```python
from build123d import *

# Parameters (mm, degrees)
ESQUISSE1_W                  = 65
ESQUISSE1_H                  = 30
BOSS_EXTRU_1_DEPTH           = 2
ESQUISSE2_R                  = 3
BOSS_EXTRU_2_DEPTH           = 8
BOSS_EXTRU_2_DRAFT           = 18
BOSS_EXTRU_2_PROFILE_2_DEPTH = 8
BOSS_EXTRU_2_PROFILE_2_DRAFT = 18
BOSS_EXTRU_2_PROFILE_3_DEPTH = 8
BOSS_EXTRU_2_PROFILE_3_DRAFT = 18
BOSS_EXTRU_2_PROFILE_4_DEPTH = 8
BOSS_EXTRU_2_PROFILE_4_DRAFT = 18
ENL_V_MAT_EXTRU_2_REACH      = 41.058
ESQUISSE4_W                  = 22.5
ESQUISSE4_H                  = 14
ENL_V_MAT_EXTRU_3_REACH      = 41.058
ESQUISSE5_R                  = 1.5
CONG_1_R                     = 2
BOSS_EXTRU_3_REACH           = 41.415
ENL_V_MAT_EXTRU_4_REACH      = 41.415
ESQUISSE7_R                  = 1.2


with BuildPart() as part:
    # Esquisse1 → Boss.-Extru.1 (new body)
    with BuildSketch(Plane.XY):
        Rectangle(ESQUISSE1_W, ESQUISSE1_H)
    extrude(amount=BOSS_EXTRU_1_DEPTH)


with BuildPart() as boss_extru_2_tool:
    # Esquisse2 → Boss.-Extru.2 (with draft: the straight prism first)
    with BuildSketch(Plane.XY.offset(8)):
        with Locations((-29, 11.5)):
            Circle(ESQUISSE2_R)
    extrude(amount=-BOSS_EXTRU_2_DEPTH)
    # Boss.-Extru.2: the draft: its side faces are tilted about the plane it starts from
    boss_extru_2_sides = [boss_extru_2_tool.faces().sort_by_distance(p)[0] for p in [
        (-32, 11.5, 4),
    ]]
    draft(boss_extru_2_sides, Plane.XY.offset(8), BOSS_EXTRU_2_DRAFT)


with BuildPart() as part_1:
    add(part.part)

    # Boss.-Extru.2: add boss_extru_2_tool
    add(boss_extru_2_tool.part)


with BuildPart() as boss_extru_2_profile_2_tool:
    # Esquisse2 → Boss.-Extru.2 profile 2 (with draft: the straight prism first)
    with BuildSketch(Plane.XY.offset(8)):
        with Locations((29, 11.5)):
            Circle(ESQUISSE2_R)
    extrude(amount=-BOSS_EXTRU_2_PROFILE_2_DEPTH)
    # Boss.-Extru.2 profile 2: the draft: its side faces are tilted about the plane it starts from
    boss_extru_2_profile_2_sides = [boss_extru_2_profile_2_tool.faces().sort_by_distance(p)[0] for p in [
        (26, 11.5, 4),
    ]]
    draft(boss_extru_2_profile_2_sides, Plane.XY.offset(8), BOSS_EXTRU_2_PROFILE_2_DRAFT)


with BuildPart() as part_2:
    add(part_1.part)

    # Boss.-Extru.2 profile 2: add boss_extru_2_profile_2_tool
    add(boss_extru_2_profile_2_tool.part)


with BuildPart() as boss_extru_2_profile_3_tool:
    # Esquisse2 → Boss.-Extru.2 profile 3 (with draft: the straight prism first)
    with BuildSketch(Plane.XY.offset(8)):
        with Locations((29, -11.5)):
            Circle(ESQUISSE2_R)
    extrude(amount=-BOSS_EXTRU_2_PROFILE_3_DEPTH)
    # Boss.-Extru.2 profile 3: the draft: its side faces are tilted about the plane it starts from
    boss_extru_2_profile_3_sides = [boss_extru_2_profile_3_tool.faces().sort_by_distance(p)[0] for p in [
        (26, -11.5, 4),
    ]]
    draft(boss_extru_2_profile_3_sides, Plane.XY.offset(8), BOSS_EXTRU_2_PROFILE_3_DRAFT)


with BuildPart() as part_3:
    add(part_2.part)

    # Boss.-Extru.2 profile 3: add boss_extru_2_profile_3_tool
    add(boss_extru_2_profile_3_tool.part)


with BuildPart() as boss_extru_2_profile_4_tool:
    # Esquisse2 → Boss.-Extru.2 profile 4 (with draft: the straight prism first)
    with BuildSketch(Plane.XY.offset(8)):
        with Locations((-29, -11.5)):
            Circle(ESQUISSE2_R)
    extrude(amount=-BOSS_EXTRU_2_PROFILE_4_DEPTH)
    # Boss.-Extru.2 profile 4: the draft: its side faces are tilted about the plane it starts from
    boss_extru_2_profile_4_sides = [boss_extru_2_profile_4_tool.faces().sort_by_distance(p)[0] for p in [
        (-32, -11.5, 4),
    ]]
    draft(boss_extru_2_profile_4_sides, Plane.XY.offset(8), BOSS_EXTRU_2_PROFILE_4_DRAFT)


with BuildPart() as part_4:
    add(part_3.part)

    # Boss.-Extru.2 profile 4: add boss_extru_2_profile_4_tool
    add(boss_extru_2_profile_4_tool.part)

    # Esquisse4 → Enlèv. mat.-Extru.2 (cut, up to next)
    with BuildSketch(Plane.XY.offset(2), mode=Mode.PRIVATE) as enl_v_mat_extru_2_sk1:
        with Locations((13.75, 0)):
            Rectangle(ESQUISSE4_W, ESQUISSE4_H)
    enl_v_mat_extru_2_tool1 = extrude(enl_v_mat_extru_2_sk1.sketch, amount=-ENL_V_MAT_EXTRU_2_REACH, mode=Mode.PRIVATE) & part_4.part
    # Esquisse4 → Enlèv. mat.-Extru.2 (cut, up to next)
    with BuildSketch(Plane.XY.offset(2), mode=Mode.PRIVATE) as enl_v_mat_extru_2_sk2:
        with Locations((-13.75, 0)):
            Rectangle(ESQUISSE4_W, ESQUISSE4_H)
    enl_v_mat_extru_2_tool2 = extrude(enl_v_mat_extru_2_sk2.sketch, amount=-ENL_V_MAT_EXTRU_2_REACH, mode=Mode.PRIVATE) & part_4.part
    add(enl_v_mat_extru_2_tool1.solids().sort_by_distance((13.75, 0, 2))[0], mode=Mode.SUBTRACT)
    add(enl_v_mat_extru_2_tool2.solids().sort_by_distance((-13.75, 0, 2))[0], mode=Mode.SUBTRACT)

    # Esquisse5 → Enlèv. mat.-Extru.3 (cut, up to next)
    with BuildSketch(Plane.XY.offset(2), mode=Mode.PRIVATE) as enl_v_mat_extru_3_sk1:
        with Locations((-28.75, 0)):
            Circle(ESQUISSE5_R)
    enl_v_mat_extru_3_tool1 = extrude(enl_v_mat_extru_3_sk1.sketch, amount=-ENL_V_MAT_EXTRU_3_REACH, mode=Mode.PRIVATE) & part_4.part
    # Esquisse5 → Enlèv. mat.-Extru.3 (cut, up to next)
    with BuildSketch(Plane.XY.offset(2), mode=Mode.PRIVATE) as enl_v_mat_extru_3_sk2:
        with Locations((0, 11)):
            Circle(ESQUISSE5_R)
    enl_v_mat_extru_3_tool2 = extrude(enl_v_mat_extru_3_sk2.sketch, amount=-ENL_V_MAT_EXTRU_3_REACH, mode=Mode.PRIVATE) & part_4.part
    # Esquisse5 → Enlèv. mat.-Extru.3 (cut, up to next)
    with BuildSketch(Plane.XY.offset(2), mode=Mode.PRIVATE) as enl_v_mat_extru_3_sk3:
        with Locations((0, -11)):
            Circle(ESQUISSE5_R)
    enl_v_mat_extru_3_tool3 = extrude(enl_v_mat_extru_3_sk3.sketch, amount=-ENL_V_MAT_EXTRU_3_REACH, mode=Mode.PRIVATE) & part_4.part
    # Esquisse5 → Enlèv. mat.-Extru.3 (cut, up to next)
    with BuildSketch(Plane.XY.offset(2), mode=Mode.PRIVATE) as enl_v_mat_extru_3_sk4:
        with Locations((28.75, 0)):
            Circle(ESQUISSE5_R)
    enl_v_mat_extru_3_tool4 = extrude(enl_v_mat_extru_3_sk4.sketch, amount=-ENL_V_MAT_EXTRU_3_REACH, mode=Mode.PRIVATE) & part_4.part
    add(enl_v_mat_extru_3_tool1.solids().sort_by_distance((-28.75, 0, 2))[0], mode=Mode.SUBTRACT)
    add(enl_v_mat_extru_3_tool2.solids().sort_by_distance((0, 11, 2))[0], mode=Mode.SUBTRACT)
    add(enl_v_mat_extru_3_tool3.solids().sort_by_distance((0, -11, 2))[0], mode=Mode.SUBTRACT)
    add(enl_v_mat_extru_3_tool4.solids().sort_by_distance((28.75, 0, 2))[0], mode=Mode.SUBTRACT)

    # Congé1
    cong_1_edges = [part_4.edges().sort_by_distance(p)[0] for p in [
        (-2.5, 7, 1),
        (-2.5, -7, 1),
        (-25, -7, 1),
        (-25, 7, 1),
        (25, 7, 1),
        (25, -7, 1),
        (2.5, -7, 1),
        (2.5, 7, 1),
    ]]
    fillet(cong_1_edges, radius=CONG_1_R)

    # Esquisse6 → Boss.-Extru.3 (add, up to next)
    with BuildSketch(Plane.XY.offset(8), mode=Mode.PRIVATE) as boss_extru_3_sk1:
        with BuildLine():
            Line((-2.5, -4), (-2.5, 4))
            ThreePointArc((-2.5, 4), (0, 6.5), (2.5, 4))
            Line((2.5, 4), (2.5, -4))
            ThreePointArc((2.5, -4), (0, -6.5), (-2.5, -4))
        make_face()
    boss_extru_3_tool1 = extrude(boss_extru_3_sk1.sketch, amount=-BOSS_EXTRU_3_REACH, mode=Mode.PRIVATE) - part_4.part
    add(boss_extru_3_tool1.solids().sort_by_distance((0, 0, 8))[0])

    # Esquisse7 → Enlèv. mat.-Extru.4 (cut, up to next)
    with BuildSketch(Plane.XY.offset(8), mode=Mode.PRIVATE) as enl_v_mat_extru_4_sk1:
        with Locations((-29, 11.5)):
            Circle(ESQUISSE7_R)
    enl_v_mat_extru_4_tool1 = extrude(enl_v_mat_extru_4_sk1.sketch, amount=-ENL_V_MAT_EXTRU_4_REACH, mode=Mode.PRIVATE) & part_4.part
    # Esquisse7 → Enlèv. mat.-Extru.4 (cut, up to next)
    with BuildSketch(Plane.XY.offset(8), mode=Mode.PRIVATE) as enl_v_mat_extru_4_sk2:
        with Locations((29, 11.5)):
            Circle(ESQUISSE7_R)
    enl_v_mat_extru_4_tool2 = extrude(enl_v_mat_extru_4_sk2.sketch, amount=-ENL_V_MAT_EXTRU_4_REACH, mode=Mode.PRIVATE) & part_4.part
    # Esquisse7 → Enlèv. mat.-Extru.4 (cut, up to next)
    with BuildSketch(Plane.XY.offset(8), mode=Mode.PRIVATE) as enl_v_mat_extru_4_sk3:
        with Locations((29, -11.5)):
            Circle(ESQUISSE7_R)
    enl_v_mat_extru_4_tool3 = extrude(enl_v_mat_extru_4_sk3.sketch, amount=-ENL_V_MAT_EXTRU_4_REACH, mode=Mode.PRIVATE) & part_4.part
    # Esquisse7 → Enlèv. mat.-Extru.4 (cut, up to next)
    with BuildSketch(Plane.XY.offset(8), mode=Mode.PRIVATE) as enl_v_mat_extru_4_sk4:
        with Locations((-29, -11.5)):
            Circle(ESQUISSE7_R)
    enl_v_mat_extru_4_tool4 = extrude(enl_v_mat_extru_4_sk4.sketch, amount=-ENL_V_MAT_EXTRU_4_REACH, mode=Mode.PRIVATE) & part_4.part
    add(enl_v_mat_extru_4_tool1.solids().sort_by_distance((-29, 11.5, 8))[0], mode=Mode.SUBTRACT)
    add(enl_v_mat_extru_4_tool2.solids().sort_by_distance((29, 11.5, 8))[0], mode=Mode.SUBTRACT)
    add(enl_v_mat_extru_4_tool3.solids().sort_by_distance((29, -11.5, 8))[0], mode=Mode.SUBTRACT)
    add(enl_v_mat_extru_4_tool4.solids().sort_by_distance((-29, -11.5, 8))[0], mode=Mode.SUBTRACT)


solid = part_4.part
```
Input: part model. Units: mm. Frame: model coordinates. A direction names the side the tool comes from. Give positions to 0.01 mm unless a question says otherwise; leave off trailing zeros. Write each loop counter-clockwise with the first axis right and the second up, starting at its lowest first coordinate (ties: lowest second). Pieces come first, ordered by that corner, then holes. Notation, with made-up numbers: (32, -11.5) - (75, -11.5) arc R26 cw to (75, 14.5) - close; hole circle Ø7 at (47.5, -37.75). An arc over 180 degrees is marked (long way). Write item = value, one per line. Start each with the question number.
1. Ray query, L1, parallel to X at y = 3, z = 1.75; L2, parallel to Y at x = 28.75, z = 1; L3, parallel to Y at x = -30, z = 3.5. Return the intervals inside material, ascending.
2. Section query B-B, the plane z = 7.25. Count the separate pieces of the cut face and the enclosed holes in it, then the cut area to 3 significant figures.
3. First-contact query: pin 1 Ø4 at (x, y) = (-29, -11.5) entering from +Z; pin 2 Ø1 at (x, z) = (-8, 1.5) entering from -Y; pin 3 Ø2.5 at (y, z) = (-1, 5.5) entering from +X; pin 4 Ø6 at (x, y) = (-25.5, -2) entering from +Z. Flat tips, straight axial feed; report the tip coordinate or a pass-through.
4. Section query A-A, the plane x = -11. Output: boundary loops of the cut face in (y, z), then the cut area to 3 significant figures.
5. Mould query, pull axis Y, two halves, no side actions, for faces 1 (the flat face through (0, 0, 8)), 2 (the flat face through (0, 15, 1)), 3 (the cylindrical face through (-3.1, -6.43, 0.99)), 4 (the flat face through (2.5, 0, 4)). Classes: released by +Y, released by -Y, zero draft, split by the parting line, or undercut.
6. Section query D-D, the plane x = -29. Output: boundary loops of the cut face in (y, z).
7. Section query C-C, the plane x = 0. Output: boundary loops of the cut face in (y, z), then the cut area to 3 significant figures.
8. Access query for faces 5 (the flat face through (29, -13, 8)), 6 (the cylindrical face through (0.1, -6.5, 5)), 7 (the flat face through (25, 0, 1)). Directions: +Z, -Z, +X, -X, +Y, -Y. A direction counts if a zero-diameter tool reaches every point of the face in a straight line with its end or side. Return the directions, or none.
Check sheet entries:
q1.L1 = -32.5 to -25, -2.5 to 2.5, 25 to 32.5
q1.L2 = -16.77 to -12.67, -10.33 to -1.5, 1.5 to 10.33, 12.67 to 16.77
q1.L3 = -15.85 to -12.16, -10.84 to -7.15, 7.15 to 10.84, 12.16 to 15.85
q2.separate_pieces = 5
q2.enclosed_holes = 4
q2.area = 174 mm2
q3.pin_1 = 8
q3.pin_2 = -15
q3.pin_3 = 2.5
q3.pin_4 = 2
q4.outline = (-15, 0) - (-7, 0) - (-7, 2) - (-15, 2) - close; (7, 0) - (15, 0) - (15, 2) - (7, 2) - close
q4.area = 32.0 mm2
q5.face_1 = zero draft
q5.face_2 = released by +Y
q5.face_3 = undercut
q5.face_4 = undercut
q6.outline = (-17.1, 0) - (-12.7, 0) - (-12.7, 8) - (-14.5, 8) - close; (-10.3, 0) - (-1.48, 0) - (-1.48, 2) - (-6.55, 2) - (-8.5, 8) - (-10.3, 8) - close; (1.48, 0) - (10.3, 0) - (10.3, 8) - (8.5, 8) - (6.55, 2) - (1.48, 2) - close; (12.7, 0) - (17.1, 0) - (14.5, 8) - (12.7, 8) - close
q7.outline = (-15, 0) - (-12.5, 0) - (-12.5, 2) - (-15, 2) - close; (-9.5, 0) - (9.5, 0) - (9.5, 2) - (6.5, 2) - (6.5, 8) - (-6.5, 8) - (-6.5, 2) - (-9.5, 2) - close; (12.5, 0) - (15, 0) - (15, 2) - (12.5, 2) - close
q7.area = 126 mm2
q8.face_5 = +Z, +X, -X, +Y, -Y
q8.face_6 = +Z, -Y
q8.face_7 = +Z, -Z
